Part model, mm, in its own coordinate system. A direction names the side the tool comes from. Coordinates: 2 decimals unless noted, no trailing zeros. Order: outer loops, then holes, each group sorted by start corner. A loop starts at its lowest first (then second) coordinate and runs counter-clockwise, first axis right, second up. Notation, with made-up numbers: M 4,33.25 L 54,33.25 A25 ccw 54,46.25 Z; hole C 25,56 d6. An arc over 180 degrees is marked long. Write item = value, one per line. Start each with the question number.
from build123d import *

# Parameters (mm, degrees)
F0_W     = 9.398
F0_H     = 38.1
F1_DEPTH = 6.096
F2_W     = 9.398
F2_H     = 3.048
F3_DEPTH = 2.286
F4_W     = 9.398
F4_H     = 1.016
F5_DEPTH = 2.286
F6_SIZE2 = 4.3994090512
F6_SIZE  = 2.54
F7_SIZE  = 2.54
F8_DEPTH = 3.81
F9_SIZE  = 2.54
F10_SIZE = 0.762


with BuildPart() as f1:
    # F0 (on Top) → F1 (new body)
    with BuildSketch(Plane.XY):
        Rectangle(F0_W, F0_H)
    extrude(amount=F1_DEPTH)

    # F2 (on face) → F3 (cut)
    with BuildSketch(Plane.XY.offset(6.096)):
        with Locations((0, 6.604)):
            Rectangle(F2_W, F2_H)
        with Locations((0, 3.556)):
            Rectangle(F2_W, F2_H)
    extrude(amount=-F3_DEPTH, mode=Mode.SUBTRACT)

    # F4 (on face) → F5 (cut)
    with BuildSketch(Plane(origin=(0, 0, 0), x_dir=(1, 0, 0), z_dir=(0, 0, -1))):
        with Locations((0, 5.588)):
            Rectangle(F4_W, F4_H)
        with Locations((0, 4.572)):
            Rectangle(F4_W, F4_H)
    extrude(amount=-F5_DEPTH, mode=Mode.SUBTRACT)

    # F6
    f6_edges = [f1.edges().sort_by_distance(p)[0] for p in [
        (0, -19.05, 0),
    ]]
    f6_side = f1.faces().sort_by_distance((0, -12.573, 0))[0]
    chamfer(f6_edges, length=F6_SIZE, length2=F6_SIZE2, reference=f6_side)

    # F7
    f7_edges = [f1.edges().sort_by_distance(p)[0] for p in [
        (0, 19.05, 6.096),
    ]]
    chamfer(f7_edges, length=F7_SIZE)

    # F8 (add): a face of the model
    f8_faces = [f1.faces().sort_by_distance(p)[0] for p in [
        (0, -8.509, 6.096),
    ]]
    extrude(f8_faces, amount=F8_DEPTH)

    # F9
    f9_edges = [f1.edges().sort_by_distance(p)[0] for p in [
        (0, 2.032, 9.906),
        (0, -19.05, 9.906),
        (-4.699, -8.509, 9.906),
        (4.699, -8.509, 9.906),
    ]]
    chamfer(f9_edges, length=F9_SIZE)

    # F10
    f10_edges = [f1.edges().sort_by_distance(p)[0] for p in [
        (0, 8.128, 6.096),
    ]]
    chamfer(f10_edges, length=F10_SIZE)


solid = f1.part
Item 1: Pull direction Y, two halves, no side cores. Call faces 1 (the flat face through (0, -11, 0)), 2 (the flat face through (-0.066, 17.762, 4.844)), 3 (the flat face through (0, 2.032, 6)): pulls with the +Y half, pulls with the -Y half, needs draft (parallel to the pull), parting line crosses it, or undercut.
Item 2: Cut at A-A, the plane z = 1.5. Write the cut outline in (x, y), and give its area (3 significant figures).
Item 3: Cut at D-D, the plane z = 8.5. Write the cut outline in (x, y) (3 decimals).
Item 4: Flat gauge pins, fed straight in: pin 1 (5 mm diameter, centred on y = 7, z = 8, fed in from +X); pin 2 (5 mm diameter, centred on x = 0.5, y = 8, fed in from +Z); pin 3 (3 mm diameter, centred on y = -10.5, z = 8, fed in from +X); pin 4 (4 mm diameter, centred on x = 2, z = 6, fed in from +Y). Where does each tip first touch, or does it go through?
Item 5: Cut at C-C, the plane y = -9. Write the cut outline in (x, z).
Item 6: Cut at B-B, the plane x = 0. Write the cut outline in (y, z).
Item 7: 3-axis set-ups, long thin cutter, end or side, ignore diameter. For faces 4 (the flat face through (-0.066, -18.044, 8.372)), 5 (the flat face through (0, 8.128, 5)), 6 (the flat face through (0, -4.064, 1)), 7 (the flat face through (0, 13, 6.096)), 8 (the flat face through (-4.699, 0, 4)): which of +Z, -Z, +X, -X, +Y, -Y reach the whole face in a straight line?
Item 8: Wall check: line 1 along Y through (x, z) = (-3.75, 6.75); line 2 along Y through (x, z) = (3.75, 4.5); line 3 along Z through (x, y) = (-1, 4). Give the ranges that are in metal, low to high. Write a range as [from, to].
Filled sheet:
q1.face_1 = needs draft
q1.face_2 = pulls with the +Y half
q1.face_3 = undercut
q2.outline = M -4.7,-17.38 L 4.7,-17.38 L 4.7,-6.1 L -4.7,-6.1 Z; M -4.7,-4.06 L 4.7,-4.06 L 4.7,19.05 L -4.7,19.05 Z
q2.area = 323 mm2
q3.outline = M -3.565,-17.916 L 3.565,-17.916 L 3.565,0.898 L -3.565,0.898 Z
q4.pin_1 = through
q4.pin_2 = 6.1
q4.pin_3 = 4.7
q4.pin_4 = 18.61
q5.outline = M -4.7,0 L 4.7,0 L 4.7,7.37 L 2.16,9.91 L -2.16,9.91 L -4.7,7.37 Z
q6.outline = M -19.05,4.4 L -16.51,0 L -6.1,0 L -6.1,2.29 L -4.06,2.29 L -4.06,0 L 19.05,0 L 19.05,3.56 L 16.51,6.1 L 8.89,6.1 L 8.13,5.33 L 8.13,3.81 L 2.03,3.81 L 2.03,7.37 L -0.51,9.91 L -16.51,9.91 L -19.05,7.37 Z
q7.face_4 = +Z, +X, -X, -Y
q7.face_5 = +Z, +X, -X
q7.face_6 = -Z, +X, -X
q7.face_7 = +Z, +X, -X, +Y
q7.face_8 = +Z, -Z, -X, +Y, -Y
q8.line_1 = [-19.05, 2.03]
q8.line_2 = [-19.05, 2.03], [8.13, 18.11]
q8.line_3 = [0, 3.81]
